from build123d import *

# Parameters (mm, degrees)
SKETCH2_W           = 45
SKETCH2_H           = 20
BOSS_EXTRUDE1_DEPTH = 25
CUT_EXTRUDE1_START  = -20
SKETCH5_W           = 45
SKETCH5_H           = 5
CUT_EXTRUDE1_DEPTH  = 15
CUT_EXTRUDE2_DEPTH  = 45
SKETCH8_W           = 38.3
SKETCH8_H           = 9.6
CUT_EXTRUDE3_DEPTH  = 10
CUT_EXTRUDE4_REACH  = 41.131
SKETCH9_W           = 19.5
SKETCH9_H           = 16.5


with BuildPart() as part:
    # Sketch2 → Boss-Extrude1 (new body)
    with BuildSketch(Plane.XY):
        Rectangle(SKETCH2_W, SKETCH2_H)
    extrude(amount=BOSS_EXTRUDE1_DEPTH)

    # Sketch5 → Cut-Extrude1 (cut)
    with BuildSketch(Plane(origin=(0, 10, 0), x_dir=(1, 0, 0), z_dir=(0, 1, 0)).offset(CUT_EXTRUDE1_START)):
        with Locations((0, -19)):
            Rectangle(SKETCH5_W, SKETCH5_H)
    extrude(amount=CUT_EXTRUDE1_DEPTH, mode=Mode.SUBTRACT)

    # Sketch7 → Cut-Extrude2 (cut)
    with BuildSketch(Plane(origin=(22.5, 0, 0), x_dir=(0, 0, -1), z_dir=(1, 0, 0))):
        Polygon((0, -10), (0, 10), (-5.381576505, 10), align=None)
    extrude(amount=-CUT_EXTRUDE2_DEPTH, mode=Mode.SUBTRACT)

    # Sketch8 → Cut-Extrude3 (cut)
    with BuildSketch(Plane(origin=(0, -0.675150911, 2.509119438), x_dir=(-1, 0, 0), z_dir=(0, 0.25983666232132585, -0.9656525818914965))):
        Rectangle(SKETCH8_W, SKETCH8_H)
    extrude(amount=-CUT_EXTRUDE3_DEPTH, mode=Mode.SUBTRACT)

    # Cut-Extrude4: up to this plane
    cut_extrude4_end = Plane(origin=(19.15, 1.361614859, 13.412861236), z_dir=(0, 0.9656525818914965, 0.25983666232132585))
    # Sketch9 → Cut-Extrude4 (cut, up to the surface)
    with BuildSketch(Plane.XZ.offset(10), mode=Mode.PRIVATE) as cut_extrude4_sk1:
        with Locations((5.75, 8.25)):
            Rectangle(SKETCH9_W, SKETCH9_H)
    cut_extrude4_tool1 = split(extrude(cut_extrude4_sk1.sketch, amount=-CUT_EXTRUDE4_REACH, mode=Mode.PRIVATE), bisect_by=cut_extrude4_end, keep=Keep.BOTH, mode=Mode.PRIVATE)
    add(cut_extrude4_tool1.solids().sort_by_distance((5.75, -10, 8.25))[0], mode=Mode.SUBTRACT)


solid = part.part
Model file for the job. Use its own axes, mm. A direction names the side the tool comes from. Coordinates: 2 decimals unless noted, no trailing zeros. Write each loop counter-clockwise with the first axis right and the second up, starting at its lowest first coordinate (ties: lowest second). Pieces come first, ordered by that corner, then holes. Notation, with made-up numbers: (84.5, 21.25) - (100.5, 21.25) arc R27 cw to (100.5, 56.25) - close; hole circle Ø1 at (-30.75, 22.5). An arc over 180 degrees is marked (long way). Write each question's results on one line, items separated by ' | '. Start each with the question number.
1) Cut at D-D (y = 3). Write the cut outline in (x, z).
2) Probe line 1 along X through (y, z) = (-9, 14.5); line 2 along X through (y, z) = (-4, 7); line 3 along Y through (x, z) = (15.5, 17.5). List the from-to ranges inside material, lowest first. Write a range as from..to.
3) Cut at B-B (y = -4.5). Write the cut outline in (x, z), then the cut area to 3 significant figures.
4) 3-axis set-ups, long thin cutter, end or side, ignore diameter. For faces 4 (the face through (0, -3, 21.5)), 5 (the face through (-4, -7, 12)), 6 (the face through (0.27, 2.27, 10.04)), 7 (the face through (-11.47, -6.59, 6.02)): which of +Z, -Z, +X, -X, +Y, -Y reach the whole face in a straight line?
5) Cut at C-C (x = -5.5). Write the cut outline in (y, z), then the cut area to 3 significant figures.
6) Flat gauge pins, fed straight in: P1, Ø4.5, axis at x = -6.5, y = -6, coming from the -Z side; P2, Ø1.5, axis at x = -10, y = -4, coming from the -Z side; P3, Ø2.5, axis at x = 5, z = 18.5, coming from the -Y side. Where does each tip first touch, or does it go through?
7) Cut at A-A (z = 3.25). Write the cut outline in (x, y), then the cut area to 3 significant figures.
8) Mould opens along Z. For faces 1 (the face through (19, -10, 8)), 2 (the face through (0, 5, 19)), 3 (the face through (0.315, 4.584, 3.924)) say: pulls with the +Z half, pulls with the -Z half, needs draft (parallel to the pull), parting line crosses it, or undercut.
Returned:
1) outline: (-22.5, 3.5) - (-19.15, 3.5) - (-19.15, 7.32) - (19.15, 7.32) - (19.15, 3.5) - (22.5, 3.5) - (22.5, 16.5) - (-22.5, 16.5) - close; (-22.5, 21.5) - (22.5, 21.5) - (22.5, 25) - (-22.5, 25) - close
2) line 1: -22.5..-4, 15.5..22.5 | line 2: -22.5..-19.15, 19.15..22.5 | line 3: 5..10
3) outline: (-22.5, 1.48) - (-19.15, 1.48) - (-19.15, 11.84) - (-4, 11.84) - (-4, 16.5) - (-22.5, 16.5) - close; (-22.5, 21.5) - (22.5, 21.5) - (22.5, 25) - (-22.5, 25) - close; (15.5, 11.84) - (19.15, 11.84) - (19.15, 1.48) - (22.5, 1.48) - (22.5, 16.5) - (15.5, 16.5) - close | area: 346 mm^2
4) face 4: +X, -X, -Y | face 5: -Z, -Y | face 6: -Z | face 7: none
5) outline: (-10, 0) - (-5.31, 1.26) - (-7.91, 10.92) - (1.36, 13.41) - (3.96, 3.76) - (10, 5.38) - (10, 25) - (-10, 25) - (-10, 21.5) - (5, 21.5) - (5, 16.5) - (-10, 16.5) - close | area: 275 mm^2
6) P1: z = 0.47 | P2: z = 11.77 | P3: y = 5
7) outline: (-22.5, -10) - (-4, -10) - (-4, -5.85) - (-19.15, -5.85) - (-19.15, 2.08) - (-22.5, 2.08) - close; (15.5, -10) - (22.5, -10) - (22.5, 2.08) - (19.15, 2.08) - (19.15, -5.85) - (15.5, -5.85) - close | area: 159 mm^2
8) face 1: needs draft | face 2: undercut | face 3: pulls with the -Z half
